Work out the finished part from the listing and answer in its coordinate system (mm). A direction names the side the tool comes from. Round coordinates to 2 decimals unless told otherwise and drop trailing zeros. Write each loop counter-clockwise with the first axis right and the second up, starting at its lowest first coordinate (ties: lowest second). Pieces come first, ordered by that corner, then holes. Notation, with made-up numbers: M 21.5,6.25 L 62.5,6.25 A22 cw 62.5,34.25 Z; hole C 65.25,-12 d3. An arc over 180 degrees is marked long. Answer in a Markdown table with one row per item.
```python
from build123d import *

# Parameters (mm, degrees)
SKETCH_1_R          = 4
SKETCH_1_R_2        = 2
EXTRUDE_1_DEPTH     = 3
SKETCH_3_W          = 3
SKETCH_3_H          = 10
EXTRUDE_4_DEPTH     = 3
SKETCH_4_R          = 2
CUT_EXTRUDE_1_DEPTH = 3


with BuildPart() as part:
    # 草图1 → 凸台-拉伸1 (new body)
    with BuildSketch(Plane.XY):
        with BuildLine():
            Line((-15, 0), (-15, -160))
            ThreePointArc((-15, -160), (0, -175), (15, -160))
            Line((15, -160), (15, 0))
            ThreePointArc((15, 0), (0, 15), (-15, 0))
        make_face()
        with Locations((0, -160)):
            Circle(SKETCH_1_R, mode=Mode.SUBTRACT)
        with Locations((-7.5, -12)):
            Circle(SKETCH_1_R_2, mode=Mode.SUBTRACT)
        with Locations((-7.5, -26)):
            Circle(SKETCH_1_R_2, mode=Mode.SUBTRACT)
        with Locations(Location((7.5, -26, 0), (0, 0, 180))):
            Circle(SKETCH_1_R_2, mode=Mode.SUBTRACT)
        with Locations(Location((7.5, -12, 0), (0, 0, 180))):
            Circle(SKETCH_1_R_2, mode=Mode.SUBTRACT)
        with BuildLine():
            Line((0, -4), (3, -4))
            ThreePointArc((3, -4), (0, 5), (-3, -4))
            Line((-3, -4), (0, -4))
        make_face(mode=Mode.SUBTRACT)
    extrude(amount=EXTRUDE_1_DEPTH)

    # 草图3 → 凸台-拉伸4 (add)
    with BuildSketch(Plane.XY.offset(3)):
        with Locations((16.5, -5)):
            Rectangle(SKETCH_3_W, SKETCH_3_H)
        with Locations((16.5, -20)):
            Rectangle(SKETCH_3_W, SKETCH_3_H)
        with Locations((16.5, -35)):
            Rectangle(SKETCH_3_W, SKETCH_3_H)
        with Locations((16.5, -50)):
            Rectangle(SKETCH_3_W, SKETCH_3_H)
        with Locations((16.5, -65)):
            Rectangle(SKETCH_3_W, SKETCH_3_H)
        with Locations((16.5, -80)):
            Rectangle(SKETCH_3_W, SKETCH_3_H)
        with Locations((16.5, -95)):
            Rectangle(SKETCH_3_W, SKETCH_3_H)
        with Locations((16.5, -110)):
            Rectangle(SKETCH_3_W, SKETCH_3_H)
        with Locations((16.5, -125)):
            Rectangle(SKETCH_3_W, SKETCH_3_H)
        with Locations((16.5, -140)):
            Rectangle(SKETCH_3_W, SKETCH_3_H)
    extrude(amount=-EXTRUDE_4_DEPTH)

    # 草图4 → 切除-拉伸1 (cut)
    with BuildSketch(Plane.XY.offset(3)):
        with Locations((0, -80)):
            Circle(SKETCH_4_R)
    extrude(amount=-CUT_EXTRUDE_1_DEPTH, mode=Mode.SUBTRACT)


solid = part.part
```
1. The part is cut by section C-C (x = 7.5). Determine the outline of the cut face in (y, z).
Calculated:
| item | result |
|---|---|
| outline | M -172.99,0 L -28,0 L -28,3 L -172.99,3 Z; M -24,0 L -14,0 L -14,3 L -24,3 Z; M -10,0 L 12.99,0 L 12.99,3 L -10,3 Z |
2. Given pin 1 (1.5 mm diameter, centred on y = -28.5, z = 1, fed in from +X); pin 2 (1.5 mm diameter, centred on x = 17, z = 2, fed in from +Y); pin 3 (3 mm diameter, centred on x = 13, y = -84.5, fed in from -Z), each flat-ended and moving along its own axis, determine where each tip first touches the part or whether it passes through.
Calculated:
| item | result |
|---|---|
| pin 1 | stops at x = 15 |
| pin 2 | stops at y = 0 |
| pin 3 | stops at z = 0 |
3. Determine the mould class of faces 1 (the flat face through (18, -80, 2)), 2 (the cylindrical face through (0, -175, 1)), 3 (the flat face through (16, -70, 2)), 4 (the flat face through (15, -43, 1)) for opening direction Y: released by +Y, released by -Y, zero draft, split by the parting line, or undercut.
Calculated:
| item | result |
|---|---|
| face 1 | zero draft |
| face 2 | released by -Y |
| face 3 | undercut |
| face 4 | undercut |
4. The part is cut by section D-D (z = 1.75). Count the separate pieces of the cut face and the enclosed holes in it, plus the area to 3 significant figures.
Calculated:
| item | result |
|---|---|
| separate pieces | 1 |
| enclosed holes | 7 |
| area | 5,620 mm² |
5. The part is cut by section B-B (y = -80). Determine the outline of the cut face in (x, z), plus the area to 3 significant figures.
Calculated:
| item | result |
|---|---|
| outline | M -15,0 L -2,0 L -2,3 L -15,3 Z; M 2,0 L 18,0 L 18,3 L 2,3 Z |
| area | 87.0 mm² |
6. The part is cut by section A-A (x = 0). Determine the outline of the cut face in (y, z).
Calculated:
| item | result |
|---|---|
| outline | M -175,0 L -164,0 L -164,3 L -175,3 Z; M -156,0 L -82,0 L -82,3 L -156,3 Z; M -78,0 L -4,0 L -4,3 L -78,3 Z; M 5,0 L 15,0 L 15,3 L 5,3 Z |
7. A tool of negligible diameter and unlimited length cuts with its end or side. For faces 5 (the flat face through (18, -65, 2)), 6 (the flat face through (0, -4, 1)), 7 (the flat face through (16, -60, 2)), from which of +Z, -Z, +X, -X, +Y, -Y can it reach the whole face along a straight path? Write none if from no direction.
Calculated:
| item | result |
|---|---|
| face 5 | +Z, -Z, +X, +Y, -Y |
| face 6 | +Z, -Z |
| face 7 | +Z, -Z, +X |
8. Consider line 1 along Y through (x, z) = (0, 1.45); line 2 along X through (y, z) = (-12.5, 1.2); line 3 along Y through (x, z) = (-7.5, 1.75). Determine where each line is inside the solid, lowest interval first. Write a range as from..to.
Calculated:
| item | result |
|---|---|
| line 1 | y = -175..-164, -156..-82, -78..-4, 5..15 |
| line 2 | x = -15..-9.44, -5.56..5.56, 9.44..15 |
| line 3 | y = -172.99..-28, -24..-14, -10..12.99 |
